The listing builds one solid part. Answer for the finished solid, in the listing's coordinates (mm). Give positions to 0.01 mm unless a question says otherwise; leave off trailing zeros. Write each loop counter-clockwise with the first axis right and the second up, starting at its lowest first coordinate (ties: lowest second). Pieces come first, ordered by that corner, then holes. Notation, with made-up numbers: (-18.75, 27) -> (-1.75, 27) arc R34 cw to (-1.75, 65) -> close; hole circle Ø8 at (45.25, -38). An arc over 180 degrees is marked (long way). Write each question's results on one line, items separated by ' | '. Start each with the question number.
Autodesk Inventor part; units mm, degrees
ref_plane "YZ Plane" through (0, 0, 0) normal (1, 0, 0) x (0, 1, 0)
ref_plane "XZ Plane" through (0, 0, 0) normal (0, 1, 0) x (-1, 0, 0)
ref_plane "XY Plane" through (0, 0, 0) normal (0, 0, 1) x (1, 0, 0)
sketch "Sketch1" plane through (0, 0, 0) normal (0, 1, 0) x (-1, 0, 0)
  line L0 (0, 0) -> (-16, 0)
  line L1 (-16, 0) -> (-16, -20.26)
  line L2 (-16, -20.26) -> (0, -20.26)
  line L3 (0, -20.26) -> (0, 0)
  circle A0 centre (-14, -18.26) radius 1.5
  circle A1 centre (-14, -2) radius 1.5
  dimension "d0" = 20.26
  dimension "d1" = 16
  dimension "d2" = 3
  dimension "d3" = 2
  dimension "d4" = 2
  dimension "d5" = 2
extrude "Extrusion1" add sketch "Sketch1" along normal blind 1.5
properties part number "IMU SENSOR"
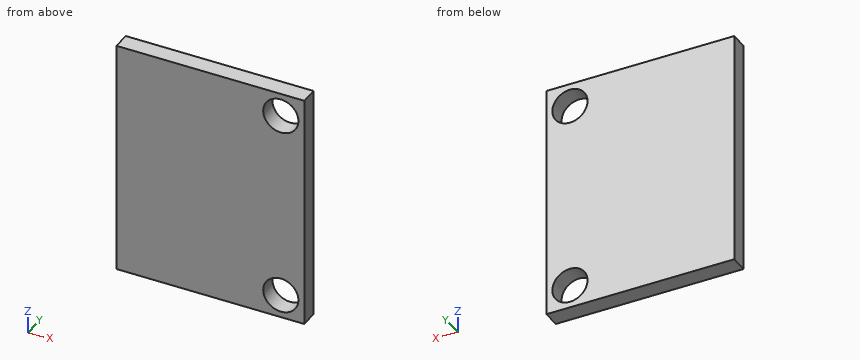
1. Consider probe 1 along Z at (x, y) = (14, 0.65); probe 2 along Z at (x, y) = (13.75, 0.4); probe 3 along X at (y, z) = (0.5, -2.75). Determine where each line is inside the solid, lowest interval first. Write a range as [from, to].
2. Section C-C (y = 0.3) is taken. Write down the section's boundary in (x, z), then the cut area to 3 significant figures.
3. Section B-B (x = 14) is taken. Write down the section's boundary in (y, z).
4. Section A-A (z = -2) is taken. Write down the section's boundary in (x, y).
Results:
1) probe 1: z = [-20.26, -19.76], [-16.76, -3.5], [-0.5, 0] | probe 2: z = [-20.26, -19.74], [-16.78, -3.48], [-0.52, 0] | probe 3: x = [0, 12.7], [15.3, 16]
2) outline: (0, -20.26) -> (16, -20.26) -> (16, 0) -> (0, 0) -> close; hole circle Ø3 at (14, -18.26); hole circle Ø3 at (14, -2) | area: 310 mm²
3) outline: (0, -20.26) -> (1.5, -20.26) -> (1.5, -19.76) -> (0, -19.76) -> close; (0, -16.76) -> (1.5, -16.76) -> (1.5, -3.5) -> (0, -3.5) -> close; (0, -0.5) -> (1.5, -0.5) -> (1.5, 0) -> (0, 0) -> close
4) outline: (0, 0) -> (12.5, 0) -> (12.5, 1.5) -> (0, 1.5) -> close; (15.5, 0) -> (16, 0) -> (16, 1.5) -> (15.5, 1.5) -> close
